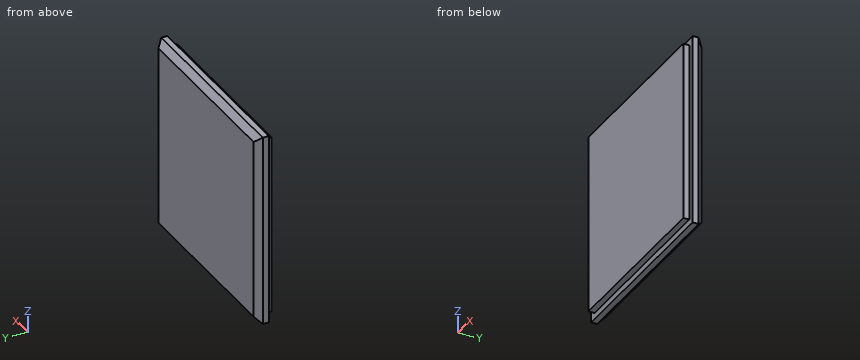
```python
from build123d import *

# Parameters (mm, degrees)
SKETCH1_W           = 101.6
SKETCH1_H           = 101.6
BOSS_EXTRUDE1_DEPTH = 9.525
SKETCH2_W           = 101.6
SKETCH2_H           = 101.6
SKETCH2_W_2         = 94.996
SKETCH2_H_2         = 94.996
CUT_EXTRUDE1_DEPTH  = 3.175
CHAMFER1_SIZE       = 3.175


with BuildPart() as part:
    # Sketch1 → Boss-Extrude1 (new body)
    with BuildSketch(Plane(origin=(0, 0, 0), x_dir=(1, 0, 0), z_dir=(0, 1, 0))):
        Rectangle(SKETCH1_W, SKETCH1_H)
    extrude(amount=BOSS_EXTRUDE1_DEPTH)

    # Sketch2 → Cut-Extrude1 (cut)
    with BuildSketch(Plane.XZ):
        Rectangle(SKETCH2_W, SKETCH2_H)
        Rectangle(SKETCH2_W_2, SKETCH2_H_2, mode=Mode.SUBTRACT)
    extrude(amount=-CUT_EXTRUDE1_DEPTH, mode=Mode.SUBTRACT)

    # Chamfer1
    chamfer1_edges = [part.edges().sort_by_distance(p)[0] for p in [
        (-50.8, 9.525, 0),
        (0, 9.525, 50.8),
        (50.8, 9.525, 0),
        (0, 9.525, -50.8),
    ]]
    chamfer(chamfer1_edges, length=CHAMFER1_SIZE)


solid = part.part
```
Design review of the part built by this model. Coordinates are the model's own, in mm. Coordinates: 2 decimals unless noted, no trailing zeros. Write each loop counter-clockwise with the first axis right and the second up, starting at its lowest first coordinate (ties: lowest second). Pieces come first, ordered by that corner, then holes.
1) Add section B-B (x = -34). Write out the cut boundary in (y, z) (3 decimals), plus the area to 3 significant figures.
2) Add section C-C (y = 8.25). Write out the cut boundary in (x, z).
3) Add section D-D (y = 2). Write out the cut boundary in (x, z).
4) Insertion check: pin 1 (2.5 mm diameter, centred on x = 9, y = 1, fed in from -Z); pin 2 (2.5 mm diameter, centred on y = 2.5, z = 12.5, fed in from -X); pin 3 (1.5 mm diameter, centred on x = 29, y = 1.5, fed in from +Z); pin 4 (1.5 mm diameter, centred on y = 1, z = 39, fed in from -X). Each pin has a flat end and moves straight along its axis. Give the tip position at first contact, or say it passes through.
5) To check wall thickness, follow L1, parallel to Z at x = -36, y = 2.75; L2, parallel to Z at x = 23, y = 7.25. State the ranges of each line that lie inside material, in increasing order.
6) Add section A-A (z = -14.5). Write out the cut boundary in (x, y) (3 decimals), plus the area to 3 significant figures.
Check result:
1. outline: (0, -47.498) - (3.175, -47.498) - (3.175, -50.8) - (6.35, -50.8) - (9.525, -47.625) - (9.525, 47.625) - (6.35, 50.8) - (3.175, 50.8) - (3.175, 47.498) - (0, 47.498) - close
1. area: 937 mm2
2. outline: (-48.9, -48.9) - (48.9, -48.9) - (48.9, 48.9) - (-48.9, 48.9) - close
3. outline: (-47.5, -47.5) - (47.5, -47.5) - (47.5, 47.5) - (-47.5, 47.5) - close
4. pin 1: stops at z = -47.5
4. pin 2: stops at x = -50.8
4. pin 3: stops at z = 47.5
4. pin 4: stops at x = -47.5
5. L1: z = -47.5 to 47.5
5. L2: z = -49.9 to 49.9
6. outline: (-50.8, 3.175) - (-47.498, 3.175) - (-47.498, 0) - (47.498, 0) - (47.498, 3.175) - (50.8, 3.175) - (50.8, 6.35) - (47.625, 9.525) - (-47.625, 9.525) - (-50.8, 6.35) - close
6. area: 937 mm2
